Verification items for this drawing (mm, ordinates from the low corner). A direction names the side the tool comes from. Coordinates: 2 decimals unless noted, no trailing zeros. Write each loop counter-clockwise with the first axis right and the second up, starting at its lowest first coordinate (ties: lowest second). Pieces come first, ordered by that corner, then holes. Notation, with made-up numbers: (79, 15.5) -> (119, 15.5) arc R24 cw to (119, 43.5) -> close; hole circle Ø11 at (-2.5, 67). An arc over 180 degrees is marked (long way). One line per question, with ' | ' between items.
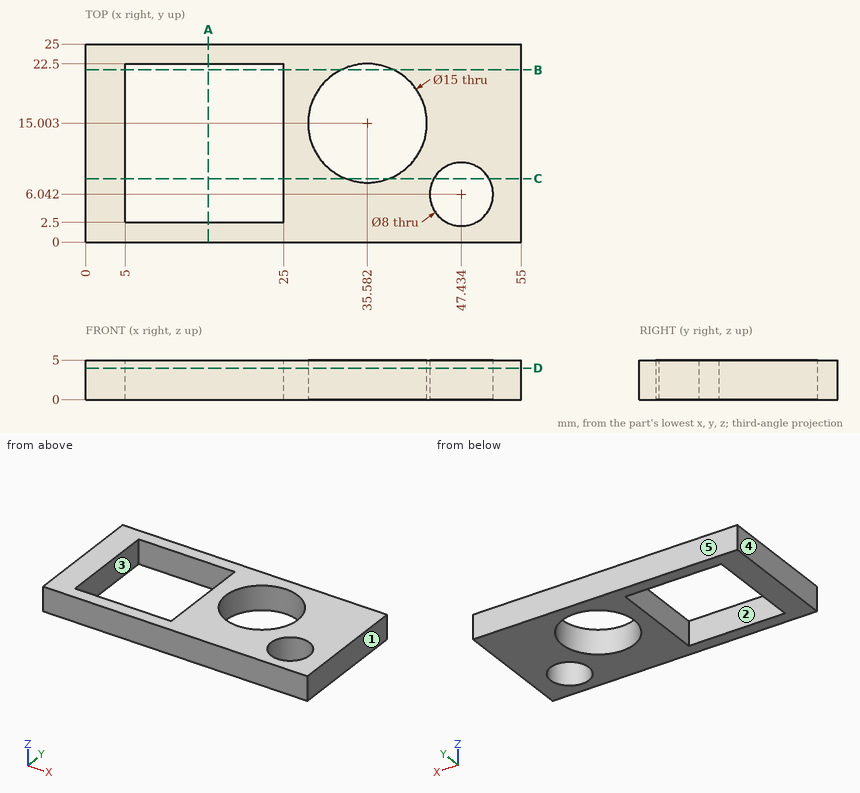
(1) Tool access check on the marked faces 1 and 2. Record the directions out of +Z, -Z, +X, -X, +Y, -Y that give a thin tool (end or side, any length) a straight path to the whole face; none if there is none.
Answers below:
face 1: +Z, -Z, +X, +Y, -Y | face 2: +Z, -Z
(2) Cross-section at C-C (y = 8). Record the cut outline in (x, z).
Answers below:
outline: (0, 0) -> (5, 0) -> (5, 5) -> (0, 5) -> close; (25, 0) -> (32.9, 0) -> (32.9, 5) -> (25, 5) -> close; (38.27, 0) -> (43.95, 0) -> (43.95, 5) -> (38.27, 5) -> close; (50.92, 0) -> (55, 0) -> (55, 5) -> (50.92, 5) -> close
(3) Cross-section at D-D (z = 4). Record the cut outline in (x, y) (1 decimal), plus the area to 3 significant figures.
Answers below:
outline: (0, 0) -> (55, 0) -> (55, 25) -> (0, 25) -> close; hole (5, 2.5) -> (25, 2.5) -> (25, 22.5) -> (5, 22.5) -> close; hole circle Ø15 at (35.6, 15); hole circle Ø8 at (47.4, 6) | area: 748 mm²
(4) Cross-section at A-A (x = 15.5). Record the cut outline in (y, z).
Answers below:
outline: (0, 0) -> (2.5, 0) -> (2.5, 5) -> (0, 5) -> close; (22.5, 0) -> (25, 0) -> (25, 5) -> (22.5, 5) -> close
(5) Draft check along X on the marked faces 3, 4 and 5. Enter one of: pulls with the +X half, pulls with the -X half, needs draft (parallel to the pull), parting line crosses it, or undercut.
Answers below:
face 3: undercut | face 4: pulls with the -X half | face 5: needs draft
(6) Material ranges on line 1 (Y direction, x = 47.5, z = 0.7); line 2 (X direction, y = 13.75, z = 2.55); line 3 (Y direction, x = 19.5, z = 2.2), recorded low to high.
Answers below:
line 1: y = 0 to 2.04, 10.04 to 25 | line 2: x = 0 to 5, 25 to 28.19, 42.98 to 55 | line 3: y = 0 to 2.5, 22.5 to 25
(7) Cross-section at B-B (y = 21.75). Record the cut outline in (x, z).
Answers below:
outline: (0, 0) -> (5, 0) -> (5, 5) -> (0, 5) -> close; (25, 0) -> (32.31, 0) -> (32.31, 5) -> (25, 5) -> close; (38.86, 0) -> (55, 0) -> (55, 5) -> (38.86, 5) -> close
